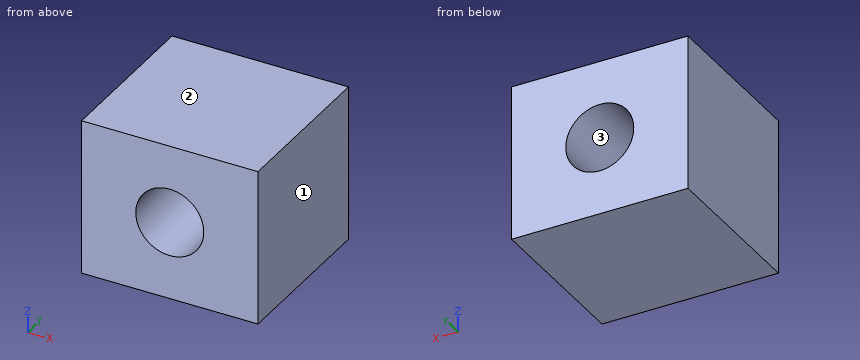
from build123d import *

# Parameters (mm, degrees)
F0_W     = 65.84879
F0_H     = 58.198094
F1_DEPTH = 60.86109
F4_D     = 25.4


with BuildPart() as f1:
    # F0 (on Front) → F1 (new body)
    with BuildSketch(Plane.XZ):
        Rectangle(F0_W, F0_H)
    extrude(amount=F1_DEPTH)

    # F4 (through all)
    with Locations(Plane.XZ.offset(60.86109)):
        with Locations((0, 0)):
            Hole(F4_D / 2)


solid = f1.part
Model file for the job. Use its own axes, mm. Face numbers are marked on the shaded views. Give positions to 0.01 mm unless a question says otherwise; leave off trailing zeros. Loops run counter-clockwise (first coordinate to the right, second up) from the corner with the lowest first, then second, coordinate; pieces in that order, holes last.
1) Saw through at B-B (z = 0). Write the cut outline in (x, y).
2) Wall check: line 1 (Z direction, x = 0, y = -23); line 2 (Z direction, x = 5, y = -12.5); line 3 (X direction, y = -27, z = -6.5). Give the ranges that are in metal, low to high.
3) Saw through at C-C (y = -20). Write the cut outline in (x, z).
4) Pull direction X, two halves, no side cores. Call the marked faces 1, 2 and 3: +X half, -X half, draft (parallel to the pull), parting line (faces both ways), or undercut.
5) Saw through at A-A (x = 0). Write the cut outline in (y, z).
Answer block:
1. outline: (-32.92, -60.86) - (-12.7, -60.86) - (-12.7, 0) - (-32.92, 0) - close; (12.7, -60.86) - (32.92, -60.86) - (32.92, 0) - (12.7, 0) - close
2. line 1: z = -29.1 to -12.7, 12.7 to 29.1
2. line 2: z = -29.1 to -11.67, 11.67 to 29.1
2. line 3: x = -32.92 to -10.91, 10.91 to 32.92
3. outline: (-32.92, -29.1) - (32.92, -29.1) - (32.92, 29.1) - (-32.92, 29.1) - close; hole circle Ø25.4 at (0, 0)
4. face 1: +X half
4. face 2: draft
4. face 3: undercut
5. outline: (-60.86, -29.1) - (0, -29.1) - (0, -12.7) - (-60.86, -12.7) - close; (-60.86, 12.7) - (0, 12.7) - (0, 29.1) - (-60.86, 29.1) - close
